Model file for the job. Use its own axes, mm. A direction names the side the tool comes from. Give positions to 0.01 mm unless a question says otherwise; leave off trailing zeros. Loops run counter-clockwise (first coordinate to the right, second up) from the corner with the lowest first, then second, coordinate; pieces in that order, holes last. Notation, with made-up numbers: M -9.75,8.25 L 38.25,8.25 A16 ccw 38.25,27.25 Z; hole C 24.25,-4 d3. An arc over 180 degrees is marked long. Answer in a Markdown table with one row per item.
```python
from build123d import *

# Parameters (mm, degrees)
F0_W      = 420
F0_H      = 420
F1_DEPTH  = 105
F2_T      = -6
F3_W      = 6
F3_H      = 408
F4_DEPTH  = 18
F5_W      = 6
F5_H      = 408
F6_DEPTH  = 18
F7_W      = 6
F7_H      = 18
F8_DEPTH  = 372
F9_W      = 6
F9_H      = 18
F10_DEPTH = 372
F11_W     = 408
F11_H     = 408
F11_W_2   = 400
F11_H_2   = 400
F12_DEPTH = 10


with BuildPart() as f1:
    # F0 (on Front) → F1 (new body, symmetric)
    with BuildSketch(Plane.XZ):
        Rectangle(F0_W, F0_H)
    extrude(amount=F1_DEPTH, both=True)

    # F2
    f2_openings = [f1.faces().sort_by_distance(p)[0] for p in [
        (0, -105, 0),
    ]]
    offset(amount=F2_T, openings=f2_openings)

    # F3 (on face) → F4 (join)
    with BuildSketch(Plane.YZ.offset(-204)):
        with Locations((-92, 0)):
            Rectangle(F3_W, F3_H)
    extrude(amount=F4_DEPTH)

    # F5 (on face) → F6 (join)
    with BuildSketch(Plane(origin=(204, 0, 0), x_dir=(0, -1, 0), z_dir=(-1, 0, 0))):
        with Locations((92, 0)):
            Rectangle(F5_W, F5_H)
    extrude(amount=F6_DEPTH)

    # F7 (on face) → F8 (join, through all)
    with BuildSketch(Plane.YZ.offset(-186)):
        with Locations((-92, 195)):
            Rectangle(F7_W, F7_H)
    extrude(amount=F8_DEPTH)

    # F9 (on face) → F10 (join, through all)
    with BuildSketch(Plane.YZ.offset(-186)):
        with Locations((-92, -195)):
            Rectangle(F9_W, F9_H)
    extrude(amount=F10_DEPTH)

    # F11 (on face) → F12 (join)
    with BuildSketch(Plane.XZ.offset(95)):
        Rectangle(F11_W, F11_H)
        Rectangle(F11_W_2, F11_H_2, mode=Mode.SUBTRACT)
    extrude(amount=F12_DEPTH)


solid = f1.part
```
Q1. 3-axis set-ups, long thin cutter, end or side, ignore diameter. For faces 4 (the face through (-17, -105, -201)), 5 (the face through (-200, -100, -3)), 6 (the face through (-3, 4, 204)): which of +Z, -Z, +X, -X, +Y, -Y reach the whole face in a straight line?
Reported:
| item | result |
|---|---|
| face 4 | +Z, -Z, +X, -X, -Y |
| face 5 | -Y |
| face 6 | none |
Q2. Saw through at A-A (y = 8.5). Give the cut face in (x, z).
Reported:
| item | result |
|---|---|
| outline | M -210,-210 L 210,-210 L 210,210 L -210,210 Z; hole M -204,-204 L 204,-204 L 204,204 L -204,204 Z |
Q3. Saw through at C-C (z = 15). Give the cut face in (x, y), and give its area (3 significant figures).
Reported:
| item | result |
|---|---|
| outline | M -210,-105 L -200,-105 L -200,-95 L -186,-95 L -186,-89 L -204,-89 L -204,99 L 204,99 L 204,-89 L 186,-89 L 186,-95 L 200,-95 L 200,-105 L 210,-105 L 210,105 L -210,105 Z |
| area | 5,260 mm² |
Q4. Drop a flat-ended pin along its axis: pin 1 (2 mm diameter, centred on x = 115.5, z = 144, fed in from -Y). Give the stop position or say it passes through.
Reported:
| item | result |
|---|---|
| pin 1 | y = 99 |
Q5. Saw through at B-B (x = 17). Give the cut face in (y, z).
Reported:
| item | result |
|---|---|
| outline | M -105,-210 L 105,-210 L 105,210 L -105,210 L -105,200 L -95,200 L -95,186 L -89,186 L -89,204 L 99,204 L 99,-204 L -89,-204 L -89,-186 L -95,-186 L -95,-200 L -105,-200 Z |
Q6. Mould opens along Z. For faces 1 (the face through (-3, 4, -204)), 2 (the face through (-210, -1, -3)), 3 (the face through (-3, -1, -210)) say: released by +Z, released by -Z, zero draft, split by the parting line, or undercut.
Reported:
| item | result |
|---|---|
| face 1 | undercut |
| face 2 | zero draft |
| face 3 | released by -Z |
Q7. Probe probe 1 along X at (y, z) = (-23, 68.5); probe 2 along Y at (x, z) = (-87, 162.5). List the from-to ranges inside material, lowest first.
Reported:
| item | result |
|---|---|
| probe 1 | -210 to -204, 204 to 210 |
| probe 2 | 99 to 105 |
